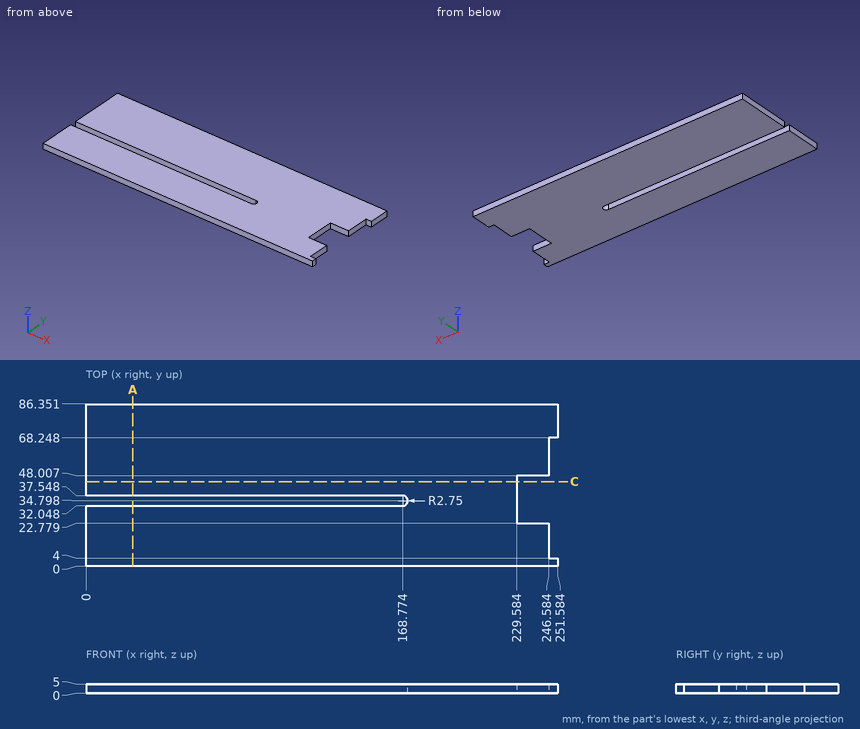
Geometry: see drawing. Coordinates: mm, zero at the bounding-box minimum. Round coordinates to 2 decimals unless told otherwise and drop trailing zeros. Write each loop counter-clockwise with the first axis right and the second up, starting at its lowest first coordinate (ties: lowest second). Pieces come first, ordered by that corner, then holes. Notation, with made-up numbers: M 83.25,65 L 141.25,65 A28 cw 141.25,93 Z; hole C 13,7 d7. An arc over 180 degrees is marked long. Answer as a JSON object with one key per item and string values. Group by question number.
(1) First-contact query: pin 1 (3 mm diameter, centred on y = 66.5, z = 2.5, fed in from +X); pin 2 (2.5 mm diameter, centred on y = 36.5, z = 2.5, fed in from +X). Flat tips, straight axial feed; report the tip coordinate or a pass-through.
(2) Ray query, line 1 (Y direction, x = 167.5, z = 3.7); line 2 (Y direction, x = 234.5, z = 4.55); line 3 (X direction, y = 45, z = 3) (1 decimal). Return the intervals inside material, ascending. Write a range as [from, to].
(3) Section query C-C on y = 45. Output: boundary loops of the cut face in (x, z) (1 decimal), then the cut area to 3 significant figures.
(4) Section query A-A on x = 25. Output: boundary loops of the cut face in (y, z).
Computed values:
{
 "1": {"pin 1": "x = 246.58", "pin 2": "x = 229.58"},
 "2": {"line 1": "[0, 32.05], [37.55, 86.35]", "line 2": "[0, 22.78], [48.01, 86.35]", "line 3": "[0, 229.6]"},
 "3": {"outline": "M 0,0 L 229.6,0 L 229.6,5 L 0,5 Z", "area": "1,150 mm^2"},
 "4": {"outline": "M 0,0 L 32.05,0 L 32.05,5 L 0,5 Z; M 37.55,0 L 86.35,0 L 86.35,5 L 37.55,5 Z"}
}
